```python
from build123d import *

# Parameters (mm, degrees)
TAP_DRILL_FOR_4_40_TAP1_D     = 2.2606
TAP_DRILL_FOR_4_40_TAP1_DEPTH = 8.89
TAP_DRILL_FOR_4_40_TAP1_TIP   = 0.679152758
TAP_DRILL_FOR_4_40_TAP2_D     = 2.2606
TAP_DRILL_FOR_4_40_TAP2_DEPTH = 8.89
TAP_DRILL_FOR_4_40_TAP2_TIP   = 0.679152758
SKETCH8_R                     = 1.524
CUT_EXTRUDE1_DEPTH            = 8.89
CIRPATTERN1_COUNT             = 6


with BuildPart() as part:
    # Sketch3 → Revolve1 (revolve)
    with BuildSketch(Plane(origin=(0, 0, 0), x_dir=(1, 0, 0), z_dir=(0, 1, 0)), mode=Mode.PRIVATE) as revolve1_sk:
        Polygon((-10, -111.125), (10, -111.125), (10, -105), (5, -105), (5, -100), (1.5875, -100), (1.5875, -100.5), (-1.5875, -100.5), (-1.5875, -100), (-5, -100), (-5, -105), (-10, -105), align=None)
    revolve(revolve1_sk.sketch.rotate(Axis((0, 0, 0), (-1, 0, 0)), 180), axis=Axis((0, 0, 0), (-1, 0, 0)))

    # Tap Drill for _4-40 Tap1
    with Locations(Plane(origin=(5, -102.5, 0), x_dir=(0, 0, 1), z_dir=(1, 0, 0))):
        with Locations((0, 0), (88.767603888, -51.25), (-88.767603888, -51.25), (-88.767603888, -153.75), (0, -205), (88.767603888, -153.75)):
            Hole(TAP_DRILL_FOR_4_40_TAP1_D / 2, depth=TAP_DRILL_FOR_4_40_TAP1_DEPTH)
            with Locations((0, 0, -(TAP_DRILL_FOR_4_40_TAP1_DEPTH + TAP_DRILL_FOR_4_40_TAP1_TIP / 2))):  # 118° drill point
                Cone(0, TAP_DRILL_FOR_4_40_TAP1_D / 2, TAP_DRILL_FOR_4_40_TAP1_TIP, mode=Mode.SUBTRACT)

    # Tap Drill for _4-40 Tap2
    with Locations(Plane(origin=(-5, -88.767603888, 51.25), x_dir=(0, 0, -1), z_dir=(-1, 0, 0))):
        with Locations((0, 0), (-51.25, -88.767603888), (0, -177.535207776), (102.5, -177.535207776), (153.75, -88.767603888), (102.5, 0)):
            Hole(TAP_DRILL_FOR_4_40_TAP2_D / 2, depth=TAP_DRILL_FOR_4_40_TAP2_DEPTH)
            with Locations((0, 0, -(TAP_DRILL_FOR_4_40_TAP2_DEPTH + TAP_DRILL_FOR_4_40_TAP2_TIP / 2))):  # 118° drill point
                Cone(0, TAP_DRILL_FOR_4_40_TAP2_D / 2, TAP_DRILL_FOR_4_40_TAP2_TIP, mode=Mode.SUBTRACT)

    # Sketch8 → Cut-Extrude1 (cut)
    with BuildSketch(Plane(origin=(0, 107.338507446, 28.761266387), x_dir=(-1, 0, 0), z_dir=(0, 0.9659258262890681, 0.25881904510252135))):
        with Locations(Location((-2.5, 0, 0), (0, 0, 90))):
            Circle(SKETCH8_R)
        with Locations(Location((2.5, 0, 0), (0, 0, 90))):
            Circle(SKETCH8_R)
    cut_extrude1 = extrude(amount=-CUT_EXTRUDE1_DEPTH, mode=Mode.SUBTRACT)

    # CirPattern1: Cut-Extrude1 ×6 about axis
    cirpattern1_axis = Axis((0, 0, 0), (1, 0, 0))
    for i in range(1, CIRPATTERN1_COUNT):
        add(cut_extrude1.rotate(cirpattern1_axis, i * 360 / CIRPATTERN1_COUNT), mode=Mode.SUBTRACT)


solid = part.part
```
Input: part model. Units: mm. Frame: model coordinates. A direction names the side the tool comes from. Give positions to 0.01 mm unless a question says otherwise; leave off trailing zeros. Order: outer loops, then holes, each group sorted by start corner. A loop starts at its lowest first (then second) coordinate and runs counter-clockwise, first axis right, second up. Notation, with made-up numbers: (87, 78.25) - (103, 78.25) arc R24 ccw to (103, 93.25) - close; hole circle Ø5 at (16.5, 60.5). An arc over 180 degrees is marked (long way). Use a Markdown table: item, result.
(1) Line query: line 1 (Y direction, x = -1, z = 0) (3 decimals); line 2 (Y direction, x = 4.1, z = 0) (3 decimals); line 3 (Z direction, x = 2.5, y = -2.5). Output: solid intervals per line, ascending. Write a range as from..to.
Computed values:
| item | result |
|---|---|
| line 1 | y = -111.125..-103.63, -101.37..-100.5, 100.5..101.37, 103.63..111.125 |
| line 2 | y = -111.125..-103.63, -101.37..-100, 100..101.37, 103.63..111.125 |
| line 3 | z = -111.1..-99.97, 99.97..111.1 |
(2) Section query A-A (y = -12.5). Output: boundary loops of the cut face in (x, z), then the cut area to 3 significant figures.
Computed values:
| item | result |
|---|---|
| outline | (-10, -110.42) - (10, -110.42) - (10, -104.25) - (5, -104.25) - (5, -99.22) - (1.59, -99.22) - (1.59, -99.72) - (-1.59, -99.72) - (-1.59, -99.22) - (-5, -99.22) - (-5, -104.25) - (-10, -104.25) - close; (-10, 104.25) - (-5, 104.25) - (-5, 99.22) - (-1.59, 99.22) - (-1.59, 99.72) - (1.59, 99.72) - (1.59, 99.22) - (5, 99.22) - (5, 104.25) - (10, 104.25) - (10, 110.42) - (-10, 110.42) - close |
| area | 344 mm2 |
(3) Pin query (flat end, axial travel): pin 1 (4 mm diameter, centred on x = -7.5, z = 24, fed in from -Y); pin 2 (1.8 mm diameter, centred on y = 51.25, z = 88.77, fed in from -X); pin 3 (1 mm diameter, centred on x = 2.5, y = -42, fed in from +Z) (3 decimals). Return the tip coordinate at first contact, or that it passes through.
Computed values:
| item | result |
|---|---|
| pin 1 | stops at y = -108.93 |
| pin 2 | stops at x = -5 |
| pin 3 | stops at z = 103.085 |
(4) Draft query along Z for faces 6 (the flat face through (10, 82, 66)), 7 (the cylindrical face through (0.14, -110.18, 14.47)), 8 (the cylindrical face through (-2.04, 102.73, 29.03)). Return one class per face: released by +Z, released by -Z, zero draft, split by the parting line, or undercut.
Computed values:
| item | result |
|---|---|
| face 6 | zero draft |
| face 7 | split by the parting line |
| face 8 | undercut |
(5) Section query B-B (z = -57.5). Output: boundary loops of the cut face in (x, y).
Computed values:
| item | result |
|---|---|
| outline | (-10, -95.09) - (10, -95.09) - (10, -87.86) - (5, -87.86) - (5, -81.82) - (1.59, -81.82) - (1.59, -82.43) - (-1.59, -82.43) - (-1.59, -81.82) - (-5, -81.82) - (-5, -87.86) - (-10, -87.86) - close; (-10, 87.86) - (-5, 87.86) - (-5, 81.82) - (-1.59, 81.82) - (-1.59, 82.43) - (1.59, 82.43) - (1.59, 81.82) - (5, 81.82) - (5, 87.86) - (10, 87.86) - (10, 95.09) - (-10, 95.09) - close |
(6) Access query for faces 1 (the cylindrical face through (-7.54, -31.54, -100.15)), 2 (the cylindrical face through (7.46, -31.54, -100.15)), 3 (the flat face through (-10, 82, -66)), 4 (the cylindrical face through (0, -68, 74)), 5 (the cylindrical face through (3.27, -30.04, -95.38)). Directions: +Z, -Z, +X, -X, +Y, -Y. A direction counts if a zero-diameter tool reaches every point of the face in a straight line with its end or side. Return the directions, or none.
Computed values:
| item | result |
|---|---|
| face 1 | -X |
| face 2 | +X |
| face 3 | +Z, -Z, -X, +Y, -Y |
| face 4 | none |
| face 5 | +X, -X |
